Here's how the part is built. I have some questions about the finished solid (model axes, mm). A direction names the side the tool comes from. Coordinates: 2 decimals unless noted, no trailing zeros. Loops run counter-clockwise (first coordinate to the right, second up) from the corner with the lowest first, then second, coordinate; pieces in that order, holes last. Notation, with made-up numbers: (68.25, 50.25) -> (93.25, 50.25) arc R20 cw to (93.25, 58.25) -> close; hole circle Ø10 at (49.25, -26.75). An arc over 180 degrees is marked (long way). Answer as a JSON object with one key per item and string values. Group by question number.
1) If we mould it in two halves opening along Y, with no side actions, what happens to faces 6 (the cylindrical face through (444.48, 97.01, 127.35)), 7 (the flat face through (444, 98.5, 122)), 8 (the flat face through (440, 78.8, 120)), 9 (the flat face through (443, 74, 122))? For each: +Y half, -Y half, draft (parallel to the pull), parting line (faces both ways), or undercut.
2) I want a section at A-A (x = 444.5). Write out the boundary of the cut face in (y, z).
3) Which directions (+Z, -Z, +X, -X, +Y, -Y) give clear straight access to the entire face, cutting with the end or side of a thin tool? Please do faces 1 (the cylindrical face through (444.48, 75.01, 127.35)), 2 (the flat face through (436, 84, 130)), 3 (the flat face through (443, 77.5, 122)), 4 (the flat face through (437, 80, 120)), 5 (the flat face through (440, 93.5, 122)).
4) I want a section at D-D (x = 438.5). Write out the boundary of the cut face in (y, z), then the cut area to 3 significant figures.
5) I'm going to push flat-ended pins straight in: pin 1 (1.9 mm diameter, centred on x = 439, z = 119, fed in from -Y); pin 2 (3 mm diameter, centred on y = 85, z = 121.5, fed in from +X); pin 3 (3 mm diameter, centred on y = 90.5, z = 117, fed in from +X); pin 4 (0.7 mm diameter, centred on x = 438.5, y = 80, fed in from -Z) (3 decimals). Where does each tip first touch, or does it pass through?
6) I need wall thicknesses on probe 1 along Y at (x, z) = (445.45, 117); probe 2 along Y at (x, z) = (444, 116.5); probe 3 along Z at (x, y) = (444.3, 74). Which ranges of each line are inside material? Lowest first, please. Write a range as [from, to].
7) I want a section at C-C (z = 120.75). Write out the boundary of the cut face in (x, y).
8) I want a section at B-B (y = 74). Write out the boundary of the cut face in (x, z), then the cut area to 3 significant figures.
```python
from build123d import *

# Parameters (mm, degrees)
CYLINDER1313_R            = 1.2
CYLINDER1313_DEPTH        = 11
CYLINDER1314_R            = 1.2
CYLINDER1314_DEPTH        = 11
CYLINDER1223_R            = 1.2
CYLINDER1223_DEPTH        = 11
CYLINDER1224_R            = 1.2
CYLINDER1224_DEPTH        = 11
BOX517_W                  = 10.4
BOX517_H                  = 12.4
BOX517_DEPTH              = 27
FILLET401_R               = 1
CYLINDER1219_R            = 8
CYLINDER1219_DEPTH        = 27
CYLINDER1221_R            = 6.5
CYLINDER1221_DEPTH        = 17
CYLINDER1220_R            = 8
CYLINDER1220_DEPTH        = 17
CYLINDER1222_R            = 8
CYLINDER1222_DEPTH        = 27
CUT014265_PLACEMENT_ANGLE = 180
BOX515_W                  = 6
BOX515_H                  = 15
BOX515_DEPTH              = 21
BOX516_W                  = 3
BOX516_H                  = 27
BOX516_DEPTH              = 16
BOX518_W                  = 12
BOX518_H                  = 17
BOX518_DEPTH              = 16
FILLET406_R               = 3
FILLET407_R               = 4


with BuildPart() as cylinder1313:
    # Cylinder1313 → Cylinder1313 (new body)
    with BuildSketch(Plane(origin=(439, 96, 121), x_dir=(0, 0, -1), z_dir=(1, 0, 0))):
        Circle(CYLINDER1313_R)
    extrude(amount=CYLINDER1313_DEPTH)


with BuildPart() as fusion248002050188:
    # Cylinder1314 → Cylinder1314 (new body)
    with BuildSketch(Plane(origin=(439, 74, 121), x_dir=(0, 0, -1), z_dir=(1, 0, 0))):
        Circle(CYLINDER1314_R)
    extrude(amount=CYLINDER1314_DEPTH)

    # Fusion248002050188: union Cylinder1313
    add(cylinder1313.part)


with BuildPart() as fusion248002050188_1:
    # Fusion248002050188 placement: moved
    add(fusion248002050188.part.moved(Location((0, 0, 7))))


with BuildPart() as cylinder1223:
    # Cylinder1223 → Cylinder1223 (new body)
    with BuildSketch(Plane(origin=(439, 96, 121), x_dir=(0, 0, -1), z_dir=(1, 0, 0))):
        Circle(CYLINDER1223_R)
    extrude(amount=CYLINDER1223_DEPTH)


with BuildPart() as fusion248002050134:
    # Cylinder1224 → Cylinder1224 (new body)
    with BuildSketch(Plane(origin=(439, 74, 121), x_dir=(0, 0, -1), z_dir=(1, 0, 0))):
        Circle(CYLINDER1224_R)
    extrude(amount=CYLINDER1224_DEPTH)

    # Fusion248002050134: union Cylinder1223
    add(cylinder1223.part)


with BuildPart() as fusion248002050134_1:
    # Fusion248002050134 placement: moved
    add(fusion248002050134.part.moved(Location((0, 0, -4))))


with BuildPart() as fillet401:
    # Box517 → Box517 (new body)
    with BuildSketch(Plane(origin=(-5.2, -6.2, 0), x_dir=(1, 0, 0), z_dir=(0, 0, 1))):
        with Locations((5.2, 6.2)):
            Rectangle(BOX517_W, BOX517_H)
    extrude(amount=BOX517_DEPTH)

    # Fillet401
    fillet401_edges = [fillet401.edges().sort_by_distance(p)[0] for p in [
        (-5.2, -6.2, 13.5),
        (-5.2, 6.2, 13.5),
        (5.2, -6.2, 13.5),
        (5.2, 6.2, 13.5),
    ]]
    fillet(fillet401_edges, radius=FILLET401_R)


with BuildPart() as cut014264:
    # Cylinder1219 → Cylinder1219 (new body)
    with BuildSketch(Plane.XY):
        Circle(CYLINDER1219_R)
    extrude(amount=CYLINDER1219_DEPTH)

    # Cut014264: cut Fillet401
    add(fillet401.part, mode=Mode.SUBTRACT)


with BuildPart() as cylinder1425:
    # Cylinder1221 → Cylinder1221 (new body)
    with BuildSketch(Plane.XY):
        Circle(CYLINDER1221_R)
    extrude(amount=CYLINDER1221_DEPTH)


with BuildPart() as fusion248002050131:
    # Cylinder1220 → Cylinder1220 (new body)
    with BuildSketch(Plane.XY):
        Circle(CYLINDER1220_R)
    extrude(amount=CYLINDER1220_DEPTH)

    # Cut014263: cut Cylinder1425
    add(cylinder1425.part, mode=Mode.SUBTRACT)

    # Fusion248002050131: union Cut014264
    add(cut014264.part)


with BuildPart() as bucket_opening_motor002:
    # Cylinder1222 → Cylinder1222 (new body)
    with BuildSketch(Plane.XY):
        Circle(CYLINDER1222_R)
    extrude(amount=CYLINDER1222_DEPTH)

    # Cut014265: cut Fusion248002050131
    add(fusion248002050131.part, mode=Mode.SUBTRACT)


with BuildPart() as bucket_opening_motor002_1:
    # Cut014265 placement: moved
    add(bucket_opening_motor002.part.moved(Location((441.5, 85, 137))).rotate(Axis((441.5, 85, 137), (1, 0, 0)), CUT014265_PLACEMENT_ANGLE))


with BuildPart() as fusion248002050132:
    # Box515 → Box515 (new body)
    with BuildSketch(Plane(origin=(441, 77.5, 109), x_dir=(1, 0, 0), z_dir=(0, 0, 1))):
        with Locations((3, 7.5)):
            Rectangle(BOX515_W, BOX515_H)
    extrude(amount=BOX515_DEPTH)

    # Fusion248002050132: union bucket-opening-motor002
    add(bucket_opening_motor002_1.part)


with BuildPart() as cube742:
    # Box516 → Box516 (new body)
    with BuildSketch(Plane(origin=(443, 71.5, 114), x_dir=(1, 0, 0), z_dir=(0, 0, 1))):
        with Locations((1.5, 13.5)):
            Rectangle(BOX516_W, BOX516_H)
    extrude(amount=BOX516_DEPTH)


with BuildPart() as bucket_opening_motor_holder:
    # Box518 → Box518 (new body)
    with BuildSketch(Plane(origin=(434, 76.5, 114), x_dir=(1, 0, 0), z_dir=(0, 0, 1))):
        with Locations((6, 8.5)):
            Rectangle(BOX518_W, BOX518_H)
    extrude(amount=BOX518_DEPTH)

    # Fusion248002050162: union Cube742
    add(cube742.part)

    # Fillet406
    fillet406_edges = [bucket_opening_motor_holder.edges().sort_by_distance(p)[0] for p in [
        (444.5, 71.5, 114),
        (444.5, 71.5, 130),
        (444.5, 98.5, 114),
        (444.5, 98.5, 130),
    ]]
    fillet(fillet406_edges, radius=FILLET406_R)

    # Fillet407
    fillet407_edges = [bucket_opening_motor_holder.edges().sort_by_distance(p)[0] for p in [
        (434, 76.5, 122),
        (434, 93.5, 122),
    ]]
    fillet(fillet407_edges, radius=FILLET407_R)

    # Cut014290: cut Fusion248002050132
    add(fusion248002050132.part, mode=Mode.SUBTRACT)

    # Cut014291: cut Fusion248002050134
    add(fusion248002050134_1.part, mode=Mode.SUBTRACT)

    # Cut014317: cut Fusion248002050188
    add(fusion248002050188_1.part, mode=Mode.SUBTRACT)


solid = bucket_opening_motor_holder.part
```
Determined:
{
 "1": {"face 6": "undercut", "face 7": "+Y half", "face 8": "undercut", "face 9": "draft"},
 "2": {"outline": "(71.5, 117) arc R3 ccw to (74.5, 114) -> (77.5, 114) -> (77.5, 130) -> (74.5, 130) arc R3 ccw to (71.5, 127) -> close; (92.5, 114) -> (95.5, 114) arc R3 ccw to (98.5, 117) -> (98.5, 127) arc R3 ccw to (95.5, 130) -> (92.5, 130) -> close; hole circle Ø2.4 at (74, 117); hole circle Ø2.4 at (74, 128); hole circle Ø2.4 at (96, 117); hole circle Ø2.4 at (96, 128)"},
 "3": {"face 1": "+X, -X", "face 2": "+Z, +X, -X, +Y, -Y", "face 3": "+Z, -Z, +X", "face 4": "-Z, +X", "face 5": "+Z, -Z, -X, +Y"},
 "4": {"outline": "(76.5, 114) -> (78.8, 114) -> (78.8, 120) -> (79.23, 120) -> (79.23, 130) -> (76.5, 130) -> close; (90.77, 120) -> (91.2, 120) -> (91.2, 114) -> (93.5, 114) -> (93.5, 130) -> (90.77, 130) -> close", "area": "82.3 mm^2"},
 "5": {"pin 1": "y = 76.5", "pin 2": "x = 436.3", "pin 3": "x = 441", "pin 4": "through"},
 "6": {"probe 1": "[71.5, 72.8], [75.2, 77.5], [92.5, 94.8], [97.2, 98.5]", "probe 2": "[71.54, 72.91], [75.09, 77.5], [92.5, 94.91], [97.09, 98.46]", "probe 3": "[114.04, 115.8], [118.2, 126.8], [129.2, 129.96]"},
 "7": {"outline": "(434, 80.5) arc R4 ccw to (438, 76.5) -> (443, 76.5) -> (443, 71.5) -> (446, 71.5) -> (446, 77.5) -> (441, 77.5) -> (441, 78.8) -> (439.55, 78.8) arc R6.5 cw to (436.3, 81.1) -> (436.3, 88.9) arc R6.5 cw to (439.55, 91.2) -> (441, 91.2) -> (441, 92.5) -> (446, 92.5) -> (446, 98.5) -> (443, 98.5) -> (443, 93.5) -> (438, 93.5) arc R4 ccw to (434, 89.5) -> close"},
 "8": {"outline": "(443, 114.04) -> (446, 114.04) -> (446, 115.8) -> (443, 115.8) -> close; (443, 118.2) -> (446, 118.2) -> (446, 126.8) -> (443, 126.8) -> close; (443, 129.2) -> (446, 129.2) -> (446, 129.96) -> (443, 129.96) -> close", "area": "33.3 mm^2"}
}
